Read the model definition and answer for the solid it produces. Units are mm, in the model's axes. Coordinates: 2 decimals unless noted, no trailing zeros. Loops run counter-clockwise (first coordinate to the right, second up) from the corner with the lowest first, then second, coordinate; pieces in that order, holes last. Notation, with made-up numbers: M 66,84 L 95,84 A25 cw 95,102 Z; hole C -26,33.25 d4. An arc over 180 degrees is marked long. One line per item, written item: value. Start each with the question number.
1. Consider probe 1 along Y at (x, z) = (18, 1.4); probe 2 along X at (y, z) = (115, 3.1); probe 3 along Y at (x, z) = (113.5, 2.2). Determine where each line is inside the solid, lowest interval first.
2. The part is cut by section A-A (x = 18). Write down the section's boundary in (y, z).
3. The part is cut by section B-B (y = 103). Write down the section's boundary in (x, z), then the cut area to 3 significant figures.
4. A flat-ended cylindrical pin translates along its axis: pin 1 (1 mm diameter, centred on x = 91, y = 132.5, fed in from -Z). Find the tip coordinate at first contact, or state that the pin passes through.
```python
from build123d import *

# Parameters (mm, degrees)
SKETCH_1_W               = 120
SKETCH_1_H               = 150
EXTRUDE_1_DEPTH          = 5
FILLET_1_R               = 10
SKETCH_2_R               = 2
CUT_EXTRUDE_1_DEPTH      = 10
MIRROR_2_COPY_1_SKETCH_R = 2
MIRROR_2_COPY_1_DEPTH    = 10


with BuildPart() as part:
    # 草图1 → 凸台-拉伸1 (new body)
    with BuildSketch(Plane.XY):
        with Locations((60, 75)):
            Rectangle(SKETCH_1_W, SKETCH_1_H)
    extrude(amount=EXTRUDE_1_DEPTH)

    # 圆角1
    fillet_1_edges = [part.edges().sort_by_distance(p)[0] for p in [
        (0, 0, 2.5),
        (0, 150, 2.5),
        (120, 150, 2.5),
        (120, 0, 2.5),
    ]]
    fillet(fillet_1_edges, radius=FILLET_1_R)

    # 草图2 → 切除-拉伸1 (cut)
    with BuildSketch(Plane.XY.offset(5)):
        with Locations((18, 47)):
            Circle(SKETCH_2_R)
        with Locations((5, 35)):
            Circle(SKETCH_2_R)
    cut_extrude_1 = extrude(amount=-CUT_EXTRUDE_1_DEPTH, mode=Mode.SUBTRACT)

    # 镜向1: 切除-拉伸1 across plane
    add(cut_extrude_1.mirror(Plane(origin=(0, 75, 0), x_dir=(0, 0, 1), z_dir=(0, -1, 0))), mode=Mode.SUBTRACT)

    # 镜向2: 切除-拉伸1 across plane
    add(cut_extrude_1.mirror(Plane.ZY.offset(-60)), mode=Mode.SUBTRACT)

    # 镜向2 copy 1 sketch → 镜向2 copy 1 (cut)
    with BuildSketch(Plane(origin=(120, 150, 5), x_dir=(-1, 0, 0), z_dir=(0, 0, 1))):
        with Locations((18, 47)):
            Circle(MIRROR_2_COPY_1_SKETCH_R)
        with Locations((5, 35)):
            Circle(MIRROR_2_COPY_1_SKETCH_R)
    extrude(amount=-MIRROR_2_COPY_1_DEPTH, mode=Mode.SUBTRACT)


solid = part.part
```
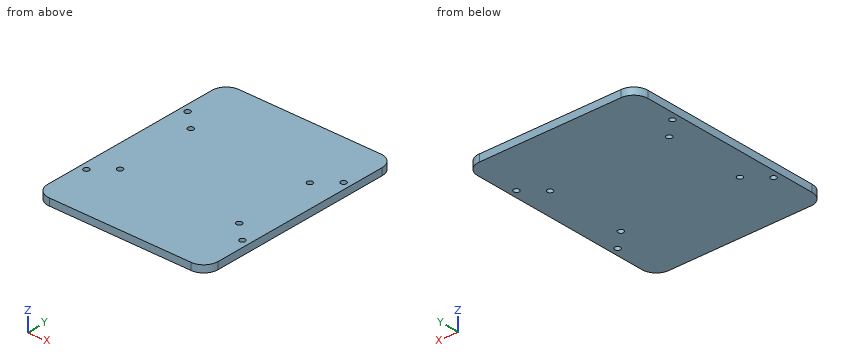
Answer block:
1. probe 1: y = 0 to 45, 49 to 101, 105 to 150
1. probe 2: x = 0 to 3, 7 to 113, 117 to 120
1. probe 3: y = 0.63 to 33.68, 36.32 to 113.68, 116.32 to 149.37
2. outline: M 0,0 L 45,0 L 45,5 L 0,5 Z; M 49,0 L 101,0 L 101,5 L 49,5 Z; M 105,0 L 150,0 L 150,5 L 105,5 Z
3. outline: M 0,0 L 16,0 L 16,5 L 0,5 Z; M 20,0 L 100,0 L 100,5 L 20,5 Z; M 104,0 L 120,0 L 120,5 L 104,5 Z
3. area: 560 mm2
4. pin 1: stops at z = 0
